CAD build for the part. Positions are in the model's coordinates, mm. Coordinates: 2 decimals unless noted, no trailing zeros. Write each loop counter-clockwise with the first axis right and the second up, starting at its lowest first coordinate (ties: lowest second). Pieces come first, ordered by that corner, then holes. Notation, with made-up numbers: M 88,26 L 126,26 A18 ccw 126,43 Z; hole C -30,29.5 d4. An arc over 180 degrees is marked long. Put each result on its own line as item: value. Start each with the question number.
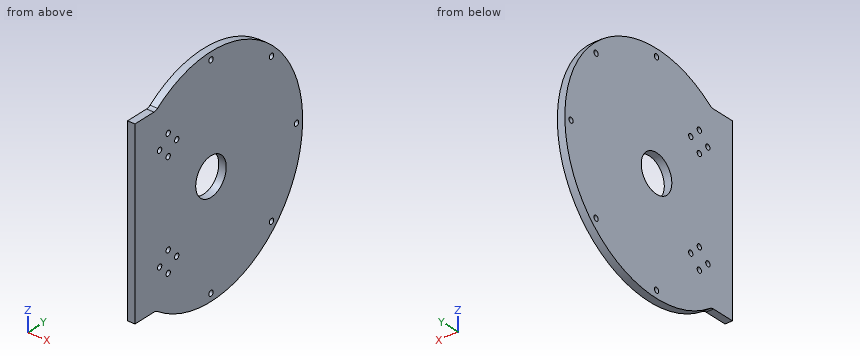
```python
from build123d import *

# Parameters (mm, degrees)
SKETCH_1_R          = 12.5
SKETCH_1_R_2        = 1.75
EXTRUDE_1_DEPTH     = 5
FILLET_1_R          = 5
SKETCH_3_R          = 1.1
CUT_EXTRUDE_2_DEPTH = 10
SKETCH_4_R          = 1.5
CUT_EXTRUDE_3_DEPTH = 10
EXTRUDE2_DEPTH      = 311.885831134
EXTRUDE2_DEPTH_BACK = 311.885831134


with BuildPart() as part:
    # 草图1 → 凸台-拉伸1 (new body)
    with BuildSketch(Plane(origin=(0, 0, 0), x_dir=(0, 0, -1), z_dir=(1, 0, 0))):
        with BuildLine():
            Line((0, 0), (0, 160))
            ThreePointArc((0, 160), (60, 280), (120, 160))
            Line((120, 160), (120, 0))
            Line((120, 0), (0, 0))
        make_face()
        with Locations((60, 205)):
            Circle(SKETCH_1_R, mode=Mode.SUBTRACT)
        with Locations((25, 177)):
            Circle(SKETCH_1_R_2, mode=Mode.SUBTRACT)
        with Locations((32, 170)):
            Circle(SKETCH_1_R_2, mode=Mode.SUBTRACT)
        with Locations((25, 163)):
            Circle(SKETCH_1_R_2, mode=Mode.SUBTRACT)
        with Locations((18, 170)):
            Circle(SKETCH_1_R_2, mode=Mode.SUBTRACT)
        with Locations((95, 177)):
            Circle(SKETCH_1_R_2, mode=Mode.SUBTRACT)
        with Locations((102, 170)):
            Circle(SKETCH_1_R_2, mode=Mode.SUBTRACT)
        with Locations((95, 163)):
            Circle(SKETCH_1_R_2, mode=Mode.SUBTRACT)
        with Locations((88, 170)):
            Circle(SKETCH_1_R_2, mode=Mode.SUBTRACT)
        with Locations((39, 140)):
            Circle(SKETCH_1_R_2, mode=Mode.SUBTRACT)
        with Locations((81, 140)):
            Circle(SKETCH_1_R_2, mode=Mode.SUBTRACT)
        with Locations((60, 275)):
            Circle(SKETCH_1_R_2, mode=Mode.SUBTRACT)
        with Locations((-10, 205)):
            Circle(SKETCH_1_R_2, mode=Mode.SUBTRACT)
        with Locations((130, 205)):
            Circle(SKETCH_1_R_2, mode=Mode.SUBTRACT)
        with Locations((10.502525317, 254.497474683)):
            Circle(SKETCH_1_R_2, mode=Mode.SUBTRACT)
        with Locations((109.497474683, 254.497474683)):
            Circle(SKETCH_1_R_2, mode=Mode.SUBTRACT)
        with Locations((5, 5)):
            Circle(SKETCH_1_R_2, mode=Mode.SUBTRACT)
        with Locations((115, 5)):
            Circle(SKETCH_1_R_2, mode=Mode.SUBTRACT)
        with Locations((5, 120)):
            Circle(SKETCH_1_R_2, mode=Mode.SUBTRACT)
        with Locations((115, 120)):
            Circle(SKETCH_1_R_2, mode=Mode.SUBTRACT)
        with BuildLine():
            Line((40.5, 81), (40.5, 59))
            ThreePointArc((40.5, 59), (39, 57.5), (37.5, 59))
            Line((37.5, 59), (37.5, 81))
            ThreePointArc((37.5, 81), (39, 82.5), (40.5, 81))
        make_face(mode=Mode.SUBTRACT)
        with BuildLine():
            Line((79.5, 81), (79.5, 59))
            ThreePointArc((79.5, 59), (81, 57.5), (82.5, 59))
            Line((82.5, 59), (82.5, 81))
            ThreePointArc((82.5, 81), (81, 82.5), (79.5, 81))
        make_face(mode=Mode.SUBTRACT)
    extrude(amount=EXTRUDE_1_DEPTH)

    # 圆角1
    fillet_1_edges = [part.edges().sort_by_distance(p)[0] for p in [
        (2.5, 0, 0),
        (2.5, 160, 0),
        (2.5, 160, -120),
        (2.5, 0, -120),
    ]]
    fillet(fillet_1_edges, radius=FILLET_1_R)

    # 草图3 → 切除-拉伸2 (cut)
    with BuildSketch(Plane.ZY):
        with Locations((-45.818141739, 127.45827935)):
            Circle(SKETCH_3_R)
        with Locations((-61.818141739, 127.45827935)):
            Circle(SKETCH_3_R)
        with Locations((-45.818141739, 91.45827935)):
            Circle(SKETCH_3_R)
        with Locations((-61.818141739, 91.45827935)):
            Circle(SKETCH_3_R)
        with BuildLine():
            Line((-20, 46.75), (-30, 46.75))
            ThreePointArc((-30, 46.75), (-31.75, 48.5), (-30, 50.25))
            Line((-30, 50.25), (-20, 50.25))
            ThreePointArc((-20, 50.25), (-18.25, 48.5), (-20, 46.75))
        make_face()
        with BuildLine():
            Line((-90, 46.75), (-100, 46.75))
            ThreePointArc((-100, 46.75), (-101.75, 48.5), (-100, 50.25))
            Line((-100, 50.25), (-90, 50.25))
            ThreePointArc((-90, 50.25), (-88.25, 48.5), (-90, 46.75))
        make_face()
        with BuildLine():
            Line((-20, 8.25), (-30, 8.25))
            ThreePointArc((-30, 8.25), (-31.75, 10), (-30, 11.75))
            Line((-30, 11.75), (-20, 11.75))
            ThreePointArc((-20, 11.75), (-18.25, 10), (-20, 8.25))
        make_face()
        with BuildLine():
            Line((-90, 8.25), (-100, 8.25))
            ThreePointArc((-100, 8.25), (-101.75, 10), (-100, 11.75))
            Line((-100, 11.75), (-90, 11.75))
            ThreePointArc((-90, 11.75), (-88.25, 10), (-90, 8.25))
        make_face()
    extrude(amount=-CUT_EXTRUDE_2_DEPTH, mode=Mode.SUBTRACT)

    # 草图4 → 切除-拉伸3 (cut)
    with BuildSketch(Plane.ZY):
        with Locations((-16.118918229, 88.740617872)):
            Circle(SKETCH_4_R)
        with Locations((-16.118918229, 64.240617872)):
            Circle(SKETCH_4_R)
        with Locations((-94, 140)):
            Circle(SKETCH_4_R)
        with Locations((-26, 140)):
            Circle(SKETCH_4_R)
        with Locations((-94, 82)):
            Circle(SKETCH_4_R)
        with Locations((-26, 82)):
            Circle(SKETCH_4_R)
    extrude(amount=-CUT_EXTRUDE_3_DEPTH, mode=Mode.SUBTRACT)

    # Sketch1 → Extrude2 (cut, two sides: drawn at the far end of the back side and taken through both)
    with BuildSketch(Plane.ZY.offset(-EXTRUDE2_DEPTH_BACK)):
        Polygon((-523.056193456, 142.822592063), (-120, 142.822592063), (0, 142.822592063), (403.056193456, 142.822592063), (403.056193456, -663.289794849), (-523.056193456, -663.289794849), align=None)
    extrude(amount=EXTRUDE2_DEPTH + EXTRUDE2_DEPTH_BACK, mode=Mode.SUBTRACT)


solid = part.part
```
(1) Drop a flat-ended pin along its axis: pin 1 (1.5 mm diameter, centred on x = 1.5, y = 264, fed in from -Z). Give the stop position or say it passes through.
(2) Slice it at C-C, the plane y = 195. Write the cut outline in (x, z).
(3) Drill centre lines: line 1 (Y direction, x = 3.4, z = -60); line 2 (Z direction, x = 4.65, y = 253); line 3 (Y direction, x = 1.2, z = -25). Where is each one in solid material? Low to high. Write a range as [from, to].
(4) Slice it at B-B, the plane y = 170. Write the cut outline in (x, z).
(5) Slice it at A-A, the plane z = -60. Write the cut outline in (x, y).
(6) Slice it at D-D, the plane x = 1.75. State how many separate pieces and enclosed holes the cut face has, then the cut area to 3 significant figures.
Result set:
1. pin 1: stops at z = -107.24
2. outline: M 0,-134.33 L 5,-134.33 L 5,-67.5 L 0,-67.5 Z; M 0,-52.5 L 5,-52.5 L 5,14.33 L 0,14.33 Z
3. line 1: y = [142.82, 192.5], [217.5, 273.25], [276.75, 280]
3. line 2: z = [-117.63, -110.4], [-108.59, -11.41], [-9.6, -2.37]
3. line 3: y = [142.82, 161.25], [164.75, 175.25], [178.75, 271.33]
4. outline: M 0,-126.33 L 5,-126.33 L 5,-103.75 L 0,-103.75 Z; M 0,-100.25 L 5,-100.25 L 5,-89.75 L 0,-89.75 Z; M 0,-86.25 L 5,-86.25 L 5,-33.75 L 0,-33.75 Z; M 0,-30.25 L 5,-30.25 L 5,-19.75 L 0,-19.75 Z; M 0,-16.25 L 5,-16.25 L 5,6.33 L 0,6.33 Z
5. outline: M 0,142.82 L 5,142.82 L 5,192.5 L 0,192.5 Z; M 0,217.5 L 5,217.5 L 5,273.25 L 0,273.25 Z; M 0,276.75 L 5,276.75 L 5,280 L 0,280 Z
6. separate pieces: 1
6. enclosed holes: 14
6. area: 16,600 mm^2
